```python
from build123d import *

# Parameters (mm, degrees)
BOSS_EXTRU_1_DEPTH       = 79.1
ESQUISSE7_W              = 7.5
ESQUISSE7_H              = 3
BOSS_EXTRU_3_DEPTH       = 36
ESQUISSE7_2_W            = 7.5
ESQUISSE7_2_H            = 3
ENL_V_MAT_EXTRU_5_DEPTH  = 36
ESQUISSE9_W              = 4
ESQUISSE9_H              = 4
BOSS_EXTRU_6_DEPTH       = 12.75
ESQUISSE11_R             = 2.5
ENL_V_MAT_EXTRU_6_DEPTH  = 10
ENL_V_START              = -5
ENL_V_MAT_EXTRU_12_DEPTH = 10
ESQUISSE13_W             = 11.5
ESQUISSE13_H             = 12
ENL_V_MAT_EXTRU_13_DEPTH = 2.5


with BuildPart() as part:
    # Esquisse1 → Boss.-Extru.1 (new body)
    with BuildSketch(Plane.XY.offset(1608.553140947)):
        with BuildLine():
            Line((0, 0), (36, 0))
            Line((36, 0), (36, 26.25))
            ThreePointArc((36, 26.25), (18, 8.25), (0, 26.25))
            Line((0, 26.25), (0, 0))
        make_face()
    extrude(amount=BOSS_EXTRU_1_DEPTH)

    # Esquisse7 → Boss.-Extru.3 (add)
    with BuildSketch(Plane(origin=(36, 0, 0), x_dir=(0, 0, -1), z_dir=(1, 0, 0))):
        with Locations((-1673.903140947, 6.5)):
            Rectangle(ESQUISSE7_W, ESQUISSE7_H)
        with Locations((-1630.303140947, 6.5)):
            Rectangle(ESQUISSE7_W, ESQUISSE7_H)
    extrude(amount=-BOSS_EXTRU_3_DEPTH)

    # Esquisse7<2> → Enlèv. mat.-Extru.5 (cut)
    with BuildSketch(Plane(origin=(36, 0, 0), x_dir=(0, 0, -1), z_dir=(1, 0, 0))):
        with Locations((-1673.903140947, 6.5)):
            Rectangle(ESQUISSE7_2_W, ESQUISSE7_2_H)
        with Locations((-1630.303140947, 6.5)):
            Rectangle(ESQUISSE7_2_W, ESQUISSE7_2_H)
    extrude(amount=-ENL_V_MAT_EXTRU_5_DEPTH, mode=Mode.SUBTRACT)

    # Esquisse9 → Boss.-Extru.6 (add)
    with BuildSketch(Plane.XZ):
        with Locations((18, 1685.653140947)):
            Rectangle(ESQUISSE9_W, ESQUISSE9_H)
    extrude(amount=-BOSS_EXTRU_6_DEPTH)

    # Esquisse11 → Enlèv. mat.-Extru.6 (cut)
    with BuildSketch(Plane.XZ):
        with Locations(Location((18, 1662.653140947, 0), (0, 0, 270))):
            Circle(ESQUISSE11_R)
        with Locations(Location((18, 1618.553140947, 0), (0, 0, 270))):
            Circle(ESQUISSE11_R)
    extrude(amount=-ENL_V_MAT_EXTRU_6_DEPTH, mode=Mode.SUBTRACT)

    # Esquisse12 → Enlèv. mat.-Extru.12 (cut)
    with BuildSketch(Plane.XZ.offset(ENL_V_START)):
        Polygon((20.309401077, 1622.553140947), (15.690598923, 1622.553140947), (13.381197846, 1618.553140947), (15.690598923, 1614.553140947), (20.309401077, 1614.553140947), (22.618802154, 1618.553140947), align=None)
        Polygon((20.309401077, 1666.653140947), (15.690598923, 1666.653140947), (13.381197846, 1662.653140947), (15.690598923, 1658.653140947), (20.309401077, 1658.653140947), (22.618802154, 1662.653140947), align=None)
    extrude(amount=-ENL_V_MAT_EXTRU_12_DEPTH, mode=Mode.SUBTRACT)

    # Esquisse13 → Enlèv. mat.-Extru.13 (cut)
    with BuildSketch(Plane.XZ):
        with Locations((30.25, 1614.553140947)):
            Rectangle(ESQUISSE13_W, ESQUISSE13_H)
        with Locations((5.75, 1614.553140947)):
            Rectangle(ESQUISSE13_W, ESQUISSE13_H)
    extrude(amount=-ENL_V_MAT_EXTRU_13_DEPTH, mode=Mode.SUBTRACT)


solid = part.part
```
Geometry: final body of the model. Coordinates: model frame, mm. A direction names the side the tool comes from. Round coordinates to 2 decimals unless told otherwise and drop trailing zeros. Write each loop counter-clockwise with the first axis right and the second up, starting at its lowest first coordinate (ties: lowest second). Pieces come first, ordered by that corner, then holes.
Item 1: Pin query (flat end, axial travel): P1, Ø0.8, axis at y = 1.5, z = 1617, coming from the +X side; P2, Ø1.2, axis at x = 18, y = 9.5, coming from the -Z side; P3, Ø8, axis at x = 12.5, z = 1675.5, coming from the +Y side. Return the tip coordinate at first contact, or that it passes through.
Item 2: Section query C-C (z = 1672.5). Return loops of the section in (x, y), plus the area to 3 significant figures.
Item 3: Section query B-B (y = 6.25). Return loops of the section in (x, z).
Item 4: Section query D-D (y = 18.5). Return loops of the section in (x, z).
Item 5: Set-up query: faces 4 (the face through (24.5, 1, 1614)), 5 (the face through (6, 1, 1620.553)), 6 (the face through (14.55, 6.9, 1620.58)), 7 (the face through (20, 11, 1686)). Return all of +Z, -Z, +X, -X, +Y, -Y with unobstructed straight access to the full face (end or side cutting, diameter ignored); none if empty.
Item 6: Material intervals for L1, parallel to Z at x = 30.5, y = 5.25; L2, parallel to Y at x = 20, z = 1650; L3, parallel to Y at x = 12.5, z = 1674, sorted ascending.
Item 7: Mould query, pull axis X, two halves, no side actions, for faces 1 (the face through (18, 6, 1677.653)), 2 (the face through (0, 13, 1648)), 3 (the face through (21.48, 6.899, 1664.625)). Classes: +X half, -X half, draft (parallel to the pull), parting line (faces both ways), or undercut.
Item 8: Section query A-A (x = 18). Give the number of separate pieces and of enclosed holes in the cut face, plus the area to 3 significant figures.
Completed:
1. P1: stops at x = 24.5
1. P2: stops at z = 1683.65
1. P3: stops at y = 10.96
2. outline: (0, 0) - (36, 0) - (36, 5) - (0, 5) - close; (0, 8) - (36, 8) - (36, 26.25) arc R18 cw to (0, 26.25) - close
2. area: 328 mm2
3. outline: (0, 1608.55) - (36, 1608.55) - (36, 1626.55) - (0, 1626.55) - close; (0, 1634.05) - (36, 1634.05) - (36, 1670.15) - (0, 1670.15) - close; (0, 1677.65) - (36, 1677.65) - (36, 1687.65) - (0, 1687.65) - close; hole (13.38, 1618.55) - (15.69, 1614.55) - (20.31, 1614.55) - (22.62, 1618.55) - (20.31, 1622.55) - (15.69, 1622.55) - close; hole (13.38, 1662.65) - (15.69, 1658.65) - (20.31, 1658.65) - (22.62, 1662.65) - (20.31, 1666.65) - (15.69, 1666.65) - close
4. outline: (0, 1608.55) - (1.75, 1608.55) - (1.75, 1687.65) - (0, 1687.65) - close; (34.25, 1608.55) - (36, 1608.55) - (36, 1687.65) - (34.25, 1687.65) - close
5. face 4: -Z, +X, -Y
5. face 5: -Z, -X, -Y
5. face 6: +Y
5. face 7: +Z, -Z, +Y
6. L1: z = 1608.55 to 1626.55, 1634.05 to 1670.15, 1677.65 to 1687.65
6. L2: y = 0 to 8.36
6. L3: y = 0 to 5, 8 to 9.11
7. face 1: draft
7. face 2: -X half
7. face 3: undercut
8. separate pieces: 3
8. enclosed holes: 2
8. area: 524 mm2
